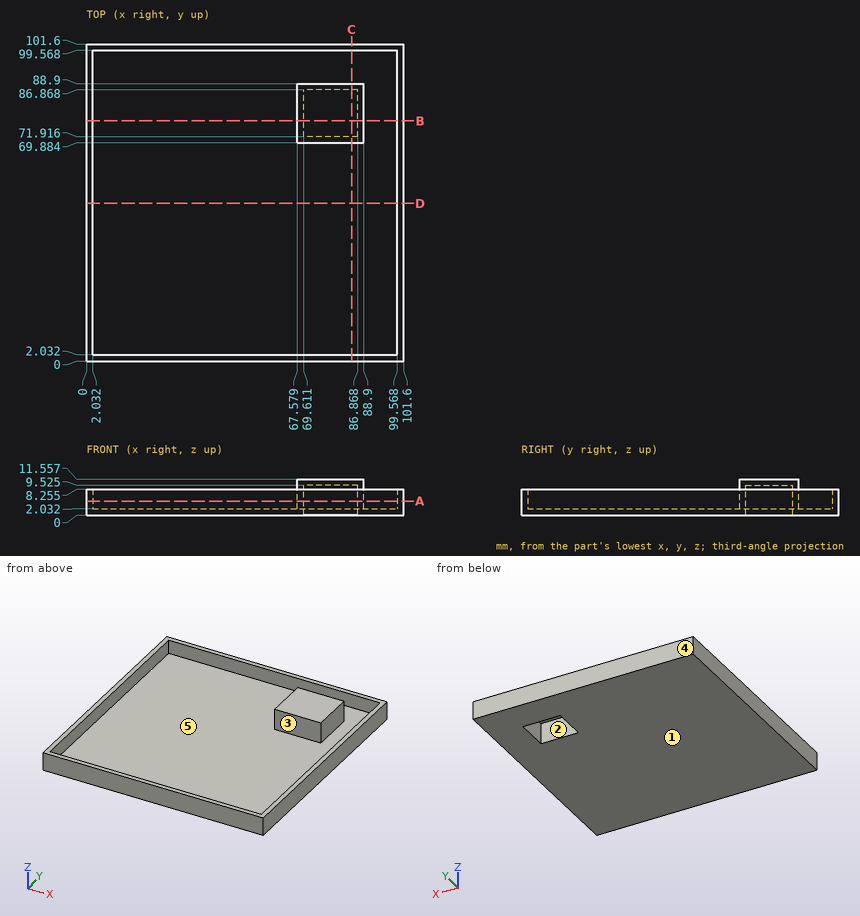
Verification items for this drawing (mm, ordinates from the low corner). A direction names the side the tool comes from. Coordinates: 2 decimals unless noted, no trailing zeros. Loops run counter-clockwise (first coordinate to the right, second up) from the corner with the lowest first, then second, coordinate; pieces in that order, holes last.
Item 1: Thickness scan on line 1 (X direction, y = 97, z = 3.75); line 2 (X direction, y = 73, z = 4). Record the ranges inside material, lowest first.
Item 2: Sectioned sample at A-A, the plane z = 4.5. Record the boundary of the cut face in (x, y) (1 decimal).
Item 3: Go/stop test with a flat-tipped pin: pin 1 Ø1 at (x, y) = (11.5, 86.5) entering from +Z. Record where the tip stops, or that it passes through.
Item 4: Release check for a two-part mould opening along X. For the marked faces 4 and 5 record: released by +X, released by -X, zero draft, split by the parting line, or undercut.
Item 5: Sectioned sample at D-D, the plane y = 50.5. Record the boundary of the cut face in (x, z) (1 decimal).
Item 6: Sectioned sample at C-C, the plane x = 85. Record the boundary of the cut face in (y, z) (1 decimal).
Item 7: Access from +Z, -Z, +X, -X, +Y, -Y to the whole of each face (thin tool, end or side, straight path). Record for the marked faces 1, 2 and 3.
Item 8: Sectioned sample at B-B, the plane y = 77. Record the boundary of the cut face in (x, z) (1 decimal).
Check result:
1. line 1: x = 0 to 2.03, 99.57 to 101.6
1. line 2: x = 0 to 2.03, 67.58 to 69.61, 86.87 to 88.9, 99.57 to 101.6
2. outline: (0, 0) - (101.6, 0) - (101.6, 101.6) - (0, 101.6) - close; (67.6, 69.9) - (88.9, 69.9) - (88.9, 88.9) - (67.6, 88.9) - close; hole (2, 2) - (99.6, 2) - (99.6, 99.6) - (2, 99.6) - close; hole (69.6, 71.9) - (86.9, 71.9) - (86.9, 86.9) - (69.6, 86.9) - close
3. pin 1: stops at z = 2.03
4. face 4: zero draft
4. face 5: undercut
5. outline: (0, 0) - (101.6, 0) - (101.6, 8.3) - (99.6, 8.3) - (99.6, 2) - (2, 2) - (2, 8.3) - (0, 8.3) - close
6. outline: (0, 0) - (71.9, 0) - (71.9, 9.5) - (86.9, 9.5) - (86.9, 0) - (101.6, 0) - (101.6, 8.3) - (99.6, 8.3) - (99.6, 2) - (88.9, 2) - (88.9, 11.6) - (69.9, 11.6) - (69.9, 2) - (2, 2) - (2, 8.3) - (0, 8.3) - close
7. face 1: -Z, +X, -X, +Y, -Y
7. face 2: -Z
7. face 3: +Z
8. outline: (0, 0) - (69.6, 0) - (69.6, 9.5) - (86.9, 9.5) - (86.9, 0) - (101.6, 0) - (101.6, 8.3) - (99.6, 8.3) - (99.6, 2) - (88.9, 2) - (88.9, 11.6) - (67.6, 11.6) - (67.6, 2) - (2, 2) - (2, 8.3) - (0, 8.3) - close
